Verification items for the finished model (mm, model axes). Face numbers are marked on the shaded views. Coordinates: 2 decimals unless noted, no trailing zeros. Order: outer loops, then holes, each group sorted by start corner. A loop starts at its lowest first (then second) coordinate and runs counter-clockwise, first axis right, second up. Notation, with made-up numbers: (18.5, -26.5) - (61.5, -26.5) arc R13 cw to (61.5, -9.5) - close; hole circle Ø8 at (3.25, 19). An arc over 180 degrees is marked (long way). Answer as CSV lines item,"result". Start each with the question number.
1. Section check B-B (y = 4). Record the cut outline in (x, z).
2. Section check A-A (x = 0). Record the cut outline in (y, z) (3 decimals), and give its area (3 significant figures).
3. Go/stop test with flat-tipped pins: pin 1 (2 mm diameter, centred on y = 2, z = 4.5, fed in from +X); pin 2 (4 mm diameter, centred on x = 3.5, z = 5.5, fed in from -Y); pin 3 (1.5 mm diameter, centred on y = 1, z = 2, fed in from -X). Record where each tip stops, or that it passes through.
4. Mould release check, pull along Z, two halves, no side actions. Record for the marked faces 1, 2, 3 and 4: pulls with the +Z half, pulls with the -Z half, needs draft (parallel to the pull), parting line crosses it, or undercut.
5. Material ranges on L1, parallel to Z at x = 0, y = 4.5; L2, parallel to X at y = 3.5, z = 1.5; L3, parallel to X at y = 5.75, z = -2, recorded low to high. Write a range as [from, to].
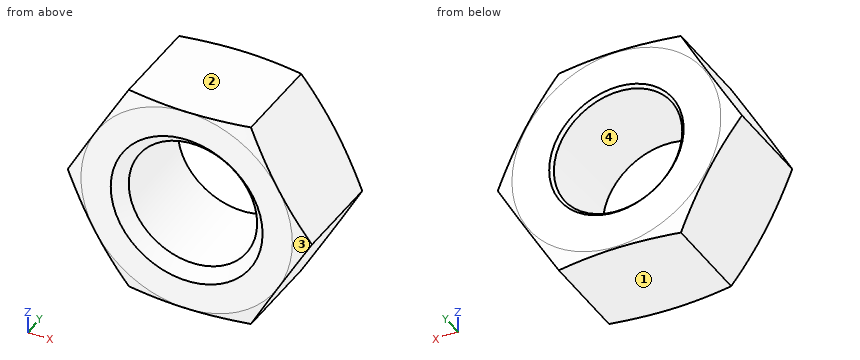
from build123d import *

# Parameters (mm, degrees)
RESSALTO_EXTRUS_O2_DEPTH         = 7
FURO_ROSCADO_DE_M101_D           = 8.5
FURO_ROSCADO_DE_M101_CSINK_D     = 10.05
FURO_ROSCADO_DE_M101_CSINK_ANGLE = 90
CHANFRO2_SIZE                    = 0.2
ESBO_O5_OUTSIDE_W                = 94.1
ESBO_O5_OUTSIDE_H                = 91.934
ESBO_O5_OUTSIDE_R                = 6.914339911
CORTE_EXTRUS_O1_DEPTH            = 13
CORTE_EXTRUS_O1_DRAFT            = -70
ESBO_O6_OUTSIDE_W                = 94.1
ESBO_O6_OUTSIDE_H                = 91.934
ESBO_O6_OUTSIDE_R                = 6.994841317
CORTE_EXTRUS_O2_DEPTH            = 13
CORTE_EXTRUS_O2_DRAFT            = -70


with BuildPart() as part:
    # Esboço1 → Ressalto-extrusão2 (new body)
    with BuildSketch(Plane(origin=(0, 0, 0), x_dir=(1, 0, 0), z_dir=(0, 1, 0))):
        Polygon((4.041451884, 7), (-4.041451884, 7), (-8.082903769, 0), (-4.041451884, -7), (4.041451884, -7), (8.082903769, 0), align=None)
    extrude(amount=RESSALTO_EXTRUS_O2_DEPTH)

    # Furo roscado de M101 (through all)
    with Locations(Plane(origin=(0, 0, 0), x_dir=(-1, 0, 0), z_dir=(0, -1, 0))):
        with Locations((0, 0)):
            CounterSinkHole(FURO_ROSCADO_DE_M101_D / 2, FURO_ROSCADO_DE_M101_CSINK_D / 2, counter_sink_angle=FURO_ROSCADO_DE_M101_CSINK_ANGLE)

    # Chanfro2
    chanfro2_edges = [part.edges().sort_by_distance(p)[0] for p in [
        (-4.25, 7, 0),
    ]]
    chamfer(chanfro2_edges, length=CHANFRO2_SIZE)


with BuildPart() as corte_extrus_o1_tool:
    # Esboço5 outside → Corte-extrusão1 (with draft: the straight prism first)
    with BuildSketch(Plane(origin=(0, 7, 0), x_dir=(1, 0, 0), z_dir=(0, 1, 0))):
        Rectangle(ESBO_O5_OUTSIDE_W, ESBO_O5_OUTSIDE_H)
        Circle(ESBO_O5_OUTSIDE_R, mode=Mode.SUBTRACT)
    extrude(amount=-CORTE_EXTRUS_O1_DEPTH)
    # Corte-extrusão1: the draft: its side faces are tilted about the plane it starts from
    corte_extrus_o1_sides = [corte_extrus_o1_tool.faces().sort_by_distance(p)[0] for p in [
        (0, 0.5, 45.967),
        (47.05, 0.5, 0),
        (0, 0.5, -45.967),
        (-47.05, 0.5, 0),
        (-6.914339911, 0.5, 0),
    ]]
    draft(corte_extrus_o1_sides, Plane(origin=(0, 7, 0), x_dir=(1, 0, 0), z_dir=(0, 1, 0)), CORTE_EXTRUS_O1_DRAFT)


with BuildPart() as part_1:
    add(part.part)

    # Corte-extrusão1: cut by corte_extrus_o1_tool
    add(corte_extrus_o1_tool.part, mode=Mode.SUBTRACT)


with BuildPart() as corte_extrus_o2_tool:
    # Esboço6 outside → Corte-extrusão2 (with draft: the straight prism first)
    with BuildSketch(Plane.XZ):
        Rectangle(ESBO_O6_OUTSIDE_W, ESBO_O6_OUTSIDE_H)
        Circle(ESBO_O6_OUTSIDE_R, mode=Mode.SUBTRACT)
    extrude(amount=-CORTE_EXTRUS_O2_DEPTH)
    # Corte-extrusão2: the draft: its side faces are tilted about the plane it starts from
    corte_extrus_o2_sides = [corte_extrus_o2_tool.faces().sort_by_distance(p)[0] for p in [
        (0, 6.5, -45.967),
        (47.05, 6.5, 0),
        (0, 6.5, 45.967),
        (-47.05, 6.5, 0),
        (-6.994841317, 6.5, 0),
    ]]
    draft(corte_extrus_o2_sides, Plane.XZ, CORTE_EXTRUS_O2_DRAFT)


with BuildPart() as part_2:
    add(part_1.part)

    # Corte-extrusão2: cut by corte_extrus_o2_tool
    add(corte_extrus_o2_tool.part, mode=Mode.SUBTRACT)


solid = part_2.part
Evaluation:
1,outline,"(-8.08, 0) - (-4.04, -7) - (4.04, -7) - (8.08, 0) - (4.04, 7) - (-4.04, 7) - close; hole circle Ø8.5 at (0, 0)"
2,outline,"(0, -6.995) - (0.002, -7) - (6.969, -7) - (7, -6.914) - (7, -4.45) - (6.8, -4.25) - (0.775, -4.25) - (0, -5.025) - close; (0, 5.025) - (0.775, 4.25) - (6.8, 4.25) - (7, 4.45) - (7, 6.914) - (6.969, 7) - (0.002, 7) - (0, 6.995) - close"
2,area,"37.9 mm²"
3,pin 1,"stops at x = 6.06"
3,pin 2,"stops at y = 0"
3,pin 3,"stops at x = -7.36"
4,face 1,"pulls with the -Z half"
4,face 2,"pulls with the +Z half"
4,face 3,"parting line crosses it"
4,face 4,"undercut"
5,L1,"z = [-7, -4.25], [4.25, 7]"
5,L2,"x = [-7.22, -3.98], [3.98, 7.22]"
5,L3,"x = [-6.93, -3.75], [3.75, 6.93]"
